Part model, mm, in its own coordinate system. Face numbers are marked on the shaded views. A direction names the side the tool comes from. Give positions to 0.01 mm unless a question says otherwise; leave off trailing zeros. Loops run counter-clockwise (first coordinate to the right, second up) from the corner with the lowest first, then second, coordinate; pieces in that order, holes last. Notation, with made-up numbers: M 67,17.25 L 112,17.25 A12 ccw 112,23.25 Z; hole C 6.25,41 d4. An arc over 180 degrees is marked long. Put each result on its own line as item: value. Start each with the question number.
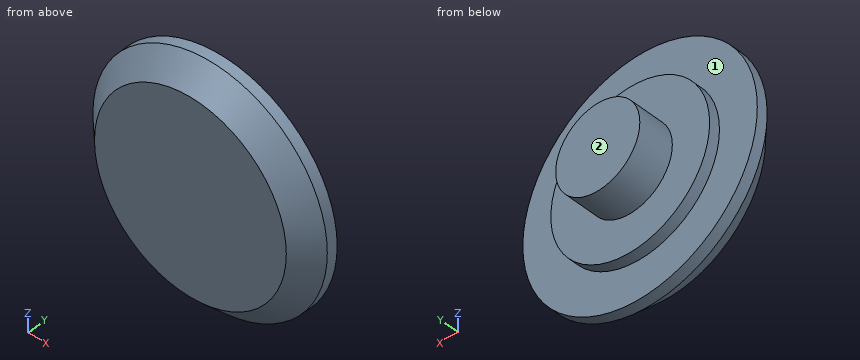
```python
from build123d import *

# Parameters (mm, degrees)
F2_SIZE = 2


with BuildPart() as f1:
    # F0 (on Top) → F1 (revolve)
    with BuildSketch(Plane.XY):
        Polygon((-11, 3), (-11, 0), (0, 0), (0, 7.3), (-3.95, 7.3), (-3.95, 4), (-7.45, 4), (-7.45, 3), align=None)
    revolve(axis=Axis((0, 3.65, 0), (0, -1, 0)))

    # F2
    f2_edges = [f1.edges().sort_by_distance(p)[0] for p in [
        (11, 0, 0),
    ]]
    chamfer(f2_edges, length=F2_SIZE)


solid = f1.part
```
1) Which spindle directions (+Z, -Z, +X, -X, +Y, -Y) get a long thin tool onto all of the face, cutting with end or side? Do the marked faces 1 and 2. Say none if no direction does.
2) Pin check, flat tips, straight feed: pin 1 Ø3 at (x, y) = (-4, 3.5) entering from -Z; pin 2 Ø2 at (x, y) = (-7.5, 1.5) entering from -Z; pin 3 Ø4 at (x, y) = (-6.5, 1) entering from +Z. Stop position of each tip, or through.
3) Band-saw the part on C-C on y = 5.5. Give the cut face in (x, z).
4) Wall check: L1, parallel to Y at x = 5.75, z = 4.25; L2, parallel to X at y = 0.75, z = -7; L3, parallel to Z at x = 4.5, y = 2.75. Give the ranges that are in metal, low to high.
5) Band-saw the part on A-A on z = 0. Give the cut face in (x, y), then the cut area to 3 significant figures.
6) Band-saw the part on B-B on x = 0. Give the cut face in (y, z).
Evaluation:
1. face 1: +Y
1. face 2: +Z, -Z, +X, -X, +Y
2. pin 1: z = -10.69
2. pin 2: z = -8.77
2. pin 3: z = 9.91
3. outline: C 0,0 d7.9
4. L1: 0 to 4
4. L2: -6.79 to 6.79
4. L3: -10.04 to 10.04
5. outline: M -11,2 L -9,0 L 9,0 L 11,2 L 11,3 L 7.45,3 L 7.45,4 L 3.95,4 L 3.95,7.3 L -3.95,7.3 L -3.95,4 L -7.45,4 L -7.45,3 L -11,3 Z
5. area: 103 mm2
6. outline: M 0,-9 L 2,-11 L 3,-11 L 3,-7.45 L 4,-7.45 L 4,-3.95 L 7.3,-3.95 L 7.3,3.95 L 4,3.95 L 4,7.45 L 3,7.45 L 3,11 L 2,11 L 0,9 Z
